Read the model definition and answer for the solid it produces. Units are mm, in the model's axes. A direction names the side the tool comes from. Give positions to 0.01 mm unless a question says otherwise; leave off trailing zeros. Write each loop counter-clockwise with the first axis right and the second up, starting at its lowest first coordinate (ties: lowest second). Pieces come first, ordered by that corner, then holes.
```python
from build123d import *

# Parameters (mm, degrees)
F0_W     = 37.973
F0_H     = 63.5
F0_W_2   = 31.7246
F0_H_2   = 57.15
F1_DEPTH = 152.4
F2_W     = 37.973
F2_H     = 63.5
F3_DEPTH = 6.35
F5_SIZE  = 2.54


with BuildPart() as f1:
    # F0 (on Front) → F1 (new body)
    with BuildSketch(Plane.XZ):
        Rectangle(F0_W, F0_H)
        Rectangle(F0_W_2, F0_H_2, mode=Mode.SUBTRACT)
    extrude(amount=F1_DEPTH)

    # F2 (on face) → F3 (join)
    with BuildSketch(Plane.XZ.offset(152.4)):
        Rectangle(F2_W, F2_H)
    extrude(amount=-F3_DEPTH)

    # F5
    f5_edges = [f1.edges().sort_by_distance(p)[0] for p in [
        (18.9865, -76.2, 31.75),
        (-18.9865, -76.2, 31.75),
        (18.9865, -76.2, -31.75),
        (-18.9865, -76.2, -31.75),
    ]]
    chamfer(f5_edges, length=F5_SIZE)


solid = f1.part
```
Item 1: Find the intervals of material crossed by line 1 along X through (y, z) = (-54, -21.5); line 2 along Z through (x, y) = (-10.5, -95) (3 decimals); line 3 along Y through (x, z) = (-5, -16.5), in increasing order.
Result set:
line 1: x = -18.99 to -15.86, 15.86 to 18.99
line 2: z = -31.75 to -28.575, 28.575 to 31.75
line 3: y = -152.4 to -146.05
Item 2: Determine the mould class of faces 3 (the flat face through (0, -75, 31.75)), 4 (the flat face through (0, -146.05, 0)), 5 (the flat face through (0, -152.4, 0)) for opening direction Z: pulls with the +Z half, pulls with the -Z half, needs draft (parallel to the pull), parting line crosses it, or undercut.
Result set:
face 3: pulls with the +Z half
face 4: undercut
face 5: needs draft
Item 3: This flat-tipped pin is pushed along its axis until it touches: pin 1 Ø2 at (x, z) = (2, 16) entering from +Y. Where does it stop, or does it pass through?
Result set:
pin 1: stops at y = -146.05
Item 4: Which of the six approach directions +Z, -Z, +X, -X, +Y, -Y give full straight-line access (tool end or side, diameter ignored) to faces 1 (the flat face through (0, -75, -31.75)), 2 (the flat face through (15.862, -72, 0))?
Result set:
face 1: -Z, +X, -X, +Y, -Y
face 2: +Y
Item 5: Section A-A (x = -11) is taken. Write down the section's boundary in (y, z) (3 decimals), and give its area (3 significant figures).
Result set:
outline: (-152.4, -31.75) - (0, -31.75) - (0, -28.575) - (-146.05, -28.575) - (-146.05, 28.575) - (0, 28.575) - (0, 31.75) - (-152.4, 31.75) - close
area: 1,330 mm2
Item 6: Section C-C (z = -22) is taken. Write down the section's boundary in (x, y).
Result set:
outline: (-18.99, -152.4) - (18.99, -152.4) - (18.99, 0) - (15.86, 0) - (15.86, -146.05) - (-15.86, -146.05) - (-15.86, 0) - (-18.99, 0) - close
